```python
from build123d import *

# Parameters (mm, degrees)
CHAMFER1_SIZE = 0.254
SCALE1_SCALE  = 1.5


with BuildPart() as part:
    # Sketch1 → Revolve1 (revolve)
    with BuildSketch(Plane.XY, mode=Mode.PRIVATE) as revolve1_sk:
        Polygon((-22.86, 0), (-22.86, 1.905), (-21.59, 1.905), (-21.59, 1.27), (21.59, 1.27), (21.59, 1.905), (22.86, 1.905), (22.86, 0), align=None)
    revolve(revolve1_sk.sketch.rotate(Axis((-22.86, 0, 0), (1, 0, 0)), 90), axis=Axis((-22.86, 0, 0), (1, 0, 0)))

    # Chamfer1
    chamfer1_edges = [part.edges().sort_by_distance(p)[0] for p in [
        (22.86, 0, -1.905),
        (-22.86, 0, -1.905),
    ]]
    chamfer(chamfer1_edges, length=CHAMFER1_SIZE)


with BuildPart() as part_1:
    # Scale1: scaled about (0, 0, 0)
    add(part.part.scale(SCALE1_SCALE))


solid = part_1.part
```
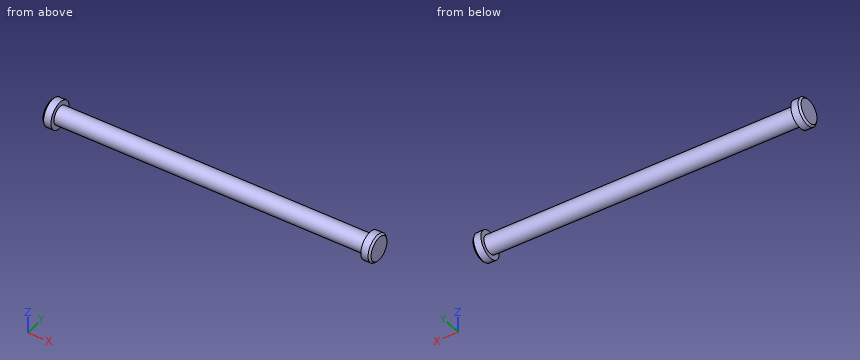
Work out the finished part from the listing and answer in its coordinate system (mm). Round coordinates to 2 decimals unless told otherwise and drop trailing zeros. Write each loop counter-clockwise with the first axis right and the second up, starting at its lowest first coordinate (ties: lowest second). Pieces come first, ordered by that corner, then holes.
1) Flat-ended cylindrical pins translate along their axes: P1, Ø3, axis at x = 25.5, z = -1, coming from the -Y side (3 decimals); P2, Ø1, axis at x = 21, z = -1.5, coming from the +Y side; P3, Ø3, axis at x = -17, y = 0, coming from the +Z side (3 decimals). Find the tip coordinate at first contact, or state that the pin passes through.
2) A cutting plane is placed at A-A on z = 0. Determine the outline of the cut face in (x, y) (1 decimal), and give its area (3 significant figures).
3) Consider probe 1 along X at (y, z) = (1.5, 1.85) (3 decimals); probe 2 along X at (y, z) = (-1.2, -2.3) (3 decimals); probe 3 along Z at (x, y) = (-12, -1.3). Determine where each line is inside the solid, lowest interval first.
4) A cutting plane is placed at C-C on x = -25.5. Determine the outline of the cut face in (y, z) (3 decimals), and give its area (3 significant figures).
Entries:
1. P1: stops at y = -1.905
1. P2: stops at y = 1.62
1. P3: stops at z = 1.905
2. outline: (-34.3, -2.5) - (-33.9, -2.9) - (-32.4, -2.9) - (-32.4, -1.9) - (32.4, -1.9) - (32.4, -2.9) - (33.9, -2.9) - (34.3, -2.5) - (34.3, 2.5) - (33.9, 2.9) - (32.4, 2.9) - (32.4, 1.9) - (-32.4, 1.9) - (-32.4, 2.9) - (-33.9, 2.9) - (-34.3, 2.5) - close
2. area: 268 mm2
3. probe 1: x = -34.29 to -32.385, 32.385 to 34.29
3. probe 2: x = -34.172 to -32.385, 32.385 to 34.172
3. probe 3: z = -1.39 to 1.39
4. outline: circle Ø3.81 at (0, 0)
4. area: 11.4 mm2
